Part print with two shaded views. Sizes in mm from the minimum x, y, z corner. A direction names the side the tool comes from. Round coordinates to 2 decimals unless told otherwise and drop trailing zeros. Loops run counter-clockwise (first coordinate to the right, second up) from the corner with the lowest first, then second, coordinate; pieces in that order, holes last. Notation, with made-up numbers: M 45.5,-8.75 L 101.5,-8.75 A30 cw 101.5,28.25 Z; hole C -3,31 d10. An arc over 180 degrees is marked long. Put each result on its own line as item: value. Start each with the question number.
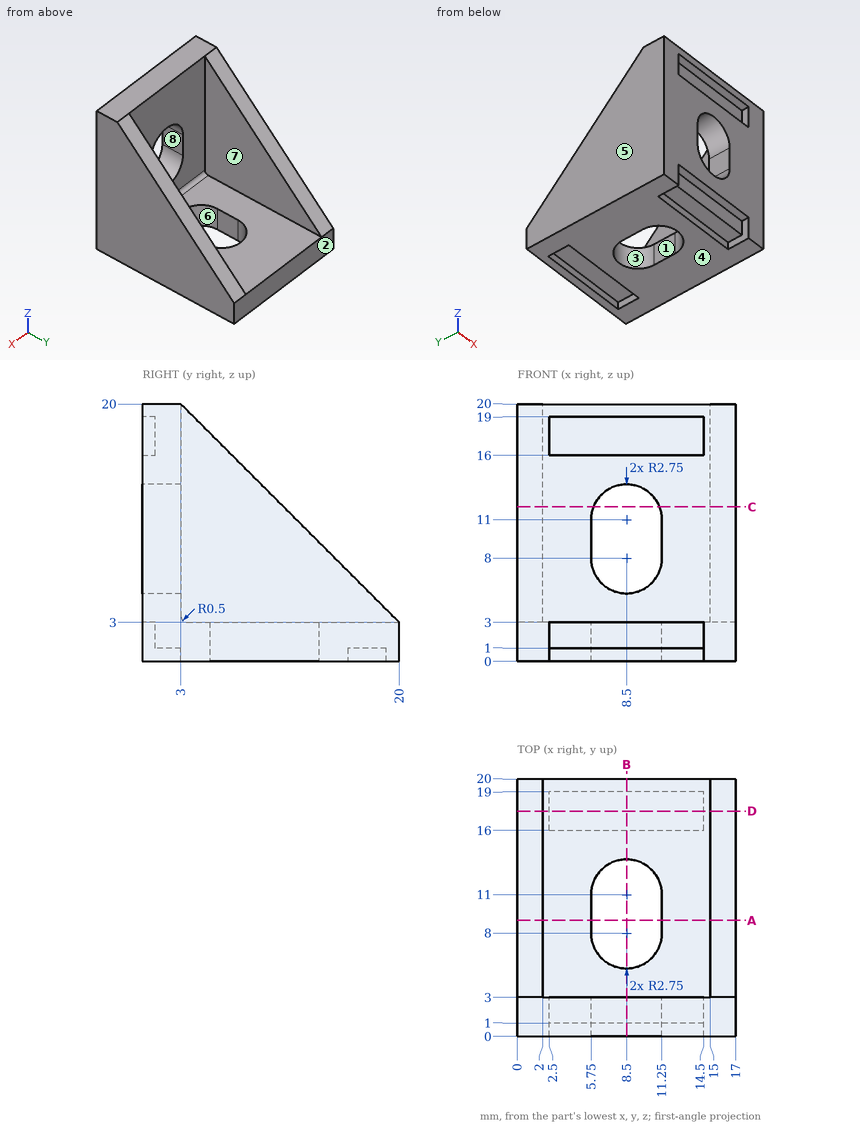
(1) Drill centre lines: line 1 along X through (y, z) = (8.5, 6.25); line 2 along X through (y, z) = (10.5, 2); line 3 along Y through (x, z) = (5.25, 10.25). Where is each one in solid material? Low to high.
(2) Mould opens along Y. For the marked faces 1, 2, 3 and 4 say: +Y half, -Y half, draft (parallel to the pull), parting line (faces both ways), or undercut.
(3) Cut at B-B on x = 8.5. List the corners of the cut face in (y, z), and give its area (3 significant figures).
(4) Tool access for the marked faces 5, 6, 7 and 8: list every direction of +Z, -Z, +X, -X, +Y, -Y with a clear straight run to the whole face (end or side of a thin tool).
(5) Flat gauge pins, fed straight in: pin 1 Ø1.5 at (x, y) = (13, 13.5) entering from +Z; pin 2 Ø0.8 at (x, y) = (6, 0.5) entering from -Z; pin 3 Ø0.9 at (x, z) = (9, 17) entering from -Y. Where does each tip first touch, or does it go through?
(6) Cut at D-D on y = 17.5. List the corners of the cut face in (x, z), and give its area (3 significant figures).
(7) Cut at A-A on y = 9. List the corners of the cut face in (x, z), and give its area (3 significant figures).
(8) Cut at C-C on z = 12. List the corners of the cut face in (x, y), and give its area (3 significant figures).
Taken from the geometry:
1. line 1: 0 to 2, 15 to 17
1. line 2: 0 to 5.75, 11.25 to 17
1. line 3: 0 to 3
2. face 1: undercut
2. face 2: +Y half
2. face 3: undercut
2. face 4: draft
3. outline: M 0,3 L 1,3 L 1,1 L 3,1 L 3,0 L 5.25,0 L 5.25,3 L 3.5,3 A0.5 cw 3,3.5 L 3,5.25 L 0,5.25 Z; M 0,13.75 L 3,13.75 L 3,20 L 0,20 L 0,19 L 1,19 L 1,16 L 0,16 Z; M 13.75,0 L 16,0 L 16,1 L 19,1 L 19,0 L 20,0 L 20,3 L 13.75,3 Z
3. area: 49.1 mm2
4. face 5: +Z, -Z, -X, +Y, -Y
4. face 6: +Z, -Z
4. face 7: +Z, +Y
4. face 8: +Y, -Y
5. pin 1: z = 3
5. pin 2: z = 3
5. pin 3: y = 1
6. outline: M 0,0 L 2.5,0 L 2.5,1 L 14.5,1 L 14.5,0 L 17,0 L 17,5.5 L 15,5.5 L 15,3 L 2,3 L 2,5.5 L 0,5.5 Z
6. area: 49.0 mm2
7. outline: M 0,0 L 5.75,0 L 5.75,3 L 2,3 L 2,14 L 0,14 Z; M 11.25,0 L 17,0 L 17,14 L 15,14 L 15,3 L 11.25,3 Z
7. area: 78.5 mm2
8. outline: M 0,0 L 5.94,0 L 5.94,3 L 2,3 L 2,11 L 0,11 Z; M 11.06,0 L 17,0 L 17,11 L 15,11 L 15,3 L 11.06,3 Z
8. area: 67.6 mm2
